```python
from build123d import *

# Parameters (mm, degrees)
SKETCH_W        = 190
SKETCH_H        = 15
PAD_DEPTH       = 5
SKETCH001_W     = 50
SKETCH001_H     = 5
PAD001_DEPTH    = 5
CHAMFER_SIZE    = 4.99
CHAMFER001_SIZE = 4.9
SKETCH002_W     = 1.482422
SKETCH002_H     = 8.21213
SKETCH002_R     = 1.233891
POCKET_DEPTH    = 1


with BuildPart() as part:
    # Sketch → Pad (new body)
    with BuildSketch(Plane.XY):
        with Locations((95, 7.5)):
            Rectangle(SKETCH_W, SKETCH_H)
    extrude(amount=PAD_DEPTH)

    # Sketch001 → Pad001 (new body)
    with BuildSketch(Plane.XY.offset(5)):
        with Locations((25, 7.5)):
            Rectangle(SKETCH001_W, SKETCH001_H)
        with Locations((165, 7.5)):
            Rectangle(SKETCH001_W, SKETCH001_H)
    extrude(amount=PAD001_DEPTH)

    # Chamfer
    chamfer_edges = [part.edges().sort_by_distance(p)[0] for p in [
        (50, 7.5, 10),
        (140, 7.5, 10),
    ]]
    chamfer(chamfer_edges, length=CHAMFER_SIZE)

    # Chamfer001
    chamfer001_edges = [part.edges().sort_by_distance(p)[0] for p in [
        (0, 7.5, 10),
        (190, 7.5, 10),
    ]]
    chamfer(chamfer001_edges, length=CHAMFER001_SIZE)

    # Sketch002 → Pocket (cut)
    with BuildSketch(Plane(origin=(0, 0, 0), x_dir=(1, 0, 0), z_dir=(0, 0, -1))):
        with Locations((35.621345, -6.948972)):
            Rectangle(SKETCH002_W, SKETCH002_H)
        Polygon((42.648026, -2.522297), (40.098263, -2.522297), (39.090214, -4.716282), (39.920372, -6.554486), (41.521393, -6.791675), (42.648026, -6.554486), (42.648026, -11.055037), (44.189751, -11.055037), (44.189751, -2.522297), align=None)
        with Locations((41.758575, -4.597689)):
            Circle(SKETCH002_R, mode=Mode.SUBTRACT)
        with BuildLine():
            add(Edge.make_bspline(
                [(48.459129, -2.517788), (43.348099, -2.730781), (46.170445, -9.027221), (48.99279, -15.323661), (51.281474, -8.814228), (53.570159, -2.304795), (48.459129, -2.517788)],
                knots=[0, 0, 0, 2.094395, 2.094395, 4.18879, 4.18879, 6.283185, 6.283185, 6.283185], degree=2, weights=[1, 0.5, 1, 0.5, 1, 0.5, 1]))
        make_face()
        with BuildLine():
            add(Edge.make_bspline(
                [(48.696312, -3.692728), (45.129949, -3.624372), (46.824186, -8.299076), (48.518424, -12.973781), (50.39055, -8.367432), (52.262675, -3.761084), (48.696312, -3.692728)],
                knots=[0, 0, 0, 2.094395, 2.094395, 4.18879, 4.18879, 6.283185, 6.283185, 6.283185], degree=2, weights=[1, 0.5, 1, 0.5, 1, 0.5, 1]))
        make_face(mode=Mode.SUBTRACT)
    extrude(amount=-POCKET_DEPTH, mode=Mode.SUBTRACT)


solid = part.part
```
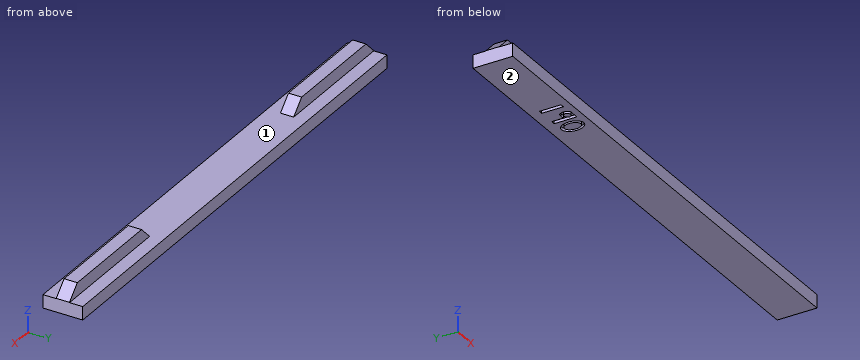
Design review of the part built by this model. Coordinates are the model's own, in mm. Face numbers are marked on the shaded views. Give positions to 0.01 mm unless a question says otherwise; leave off trailing zeros. Order: outer loops, then holes, each group sorted by start corner. A loop starts at its lowest first (then second) coordinate and runs counter-clockwise, first axis right, second up. Notation, with made-up numbers: (56, -18.75) -> (60, -18.75) arc R28 cw to (60, 19.25) -> close; hole circle Ø2 at (-3, 85). An arc over 180 degrees is marked (long way). Write each question's results on one line, items separated by ' | '. Start each with the question number.
Q1. Add section C-C on x = 99. Give the boundary of the cut face in (y, z), and give its area (3 significant figures).
Q2. Wall thickness on L1, parallel to Z at x = 60.5, y = 7.5; L2, parallel to X at y = 9.5, z = 7; L3, parallel to Y at x = 41.5, z = 9.25: over which ranges is each line inside the solid? List them lowest first. Write a range as from..to.
Q3. Add section A-A on z = 7.5. Give the boundary of the cut face in (x, y).
Q4. Mouldability with a two-part tool opening along X and no side actions: class the marked faces 1 and 2 as +X half, -X half, draft (parallel to the pull), parting line (faces both ways), or undercut.
Q5. Add section B-B on x = 159.5. Give the boundary of the cut face in (y, z), and give its area (3 significant figures).
Q6. For pin 1 (5.5 mm diameter, centred on x = 31.5, z = 8, fed in from -Y); pin 2 (1.5 mm diameter, centred on x = 111.5, y = 2.5, fed in from +Z); pin 3 (2.5 mm diameter, centred on x = 167.5, z = 7, fed in from +Y), all flat-tipped, find the tip position at first contact; note any pin that passes through.
Found:
1) outline: (0, 0) -> (15, 0) -> (15, 5) -> (0, 5) -> close | area: 75.0 mm2
2) L1: z = 0..5 | L2: x = 1.9..48.01, 141.99..188.1 | L3: y = 5..10
3) outline: (2.4, 5) -> (47.51, 5) -> (47.51, 10) -> (2.4, 10) -> close; (142.49, 5) -> (187.6, 5) -> (187.6, 10) -> (142.49, 10) -> close
4) face 1: undercut | face 2: draft
5) outline: (0, 0) -> (15, 0) -> (15, 5) -> (10, 5) -> (10, 10) -> (5, 10) -> (5, 5) -> (0, 5) -> close | area: 100 mm2
6) pin 1: stops at y = 5 | pin 2: stops at z = 5 | pin 3: stops at y = 10
